```python
from build123d import *

# Parameters (mm, degrees)
SKETCH1_R           = 13.75
BOSS_EXTRUDE1_DEPTH = 6
SHELL1_T            = -0.5
SKETCH3_R           = 5
BOSS_EXTRUDE2_DEPTH = 6
BOSS_EXTRUDE7_START = 2
SKETCH10_R          = 13.25
BOSS_EXTRUDE7_DEPTH = 2
BOSS_EXTRUDE3_START = 25.55
SKETCH4_R           = 13.75
BOSS_EXTRUDE3_DEPTH = 25.55
CHAMFER1_SIZE       = 2
SKETCH5_R           = 3.9
BOSS_EXTRUDE4_DEPTH = 4.8
SKETCH6_R           = 2.9
BOSS_EXTRUDE5_DEPTH = 4.2
CHAMFER2_SIZE       = 0.5
CUT_EXTRUDE1_START  = -5
CUT_EXTRUDE1_DEPTH  = 24.2
CUT_EXTRUDE2_START  = -5
CUT_EXTRUDE2_DEPTH  = 24.2
BOSS_EXTRUDE8_DEPTH = 6.687218579
BOSS_EXTRUDE8_DRAFT = 8


# Read off the part's stored shape, not the designer's step: Boss-Extrude8
with BuildPart() as part:
    # Sketch1 → Boss-Extrude1 (new body)
    with BuildSketch(Plane.XY):
        Circle(SKETCH1_R)
    extrude(amount=BOSS_EXTRUDE1_DEPTH)

    # Shell1
    shell1_openings = [part.faces().sort_by_distance(p)[0] for p in [
        (0, 0, 0),
    ]]
    offset(amount=SHELL1_T, openings=shell1_openings, kind=Kind.INTERSECTION)

    # Sketch3 → Boss-Extrude2 (add)
    with BuildSketch(Plane(origin=(0, 0, 5.5), x_dir=(-1, 0, 0), z_dir=(0, 0, -1))):
        with Locations(Location((0, 0, 0), (0, 0, 180))):
            Circle(SKETCH3_R)
    extrude(amount=BOSS_EXTRUDE2_DEPTH)

    # Sketch10 → Boss-Extrude7 (add)
    with BuildSketch(Plane(origin=(0, 0, 5.5), x_dir=(-1, 0, 0), z_dir=(0, 0, -1)).offset(BOSS_EXTRUDE7_START)):
        Circle(SKETCH10_R)
    extrude(amount=-BOSS_EXTRUDE7_DEPTH)

    # Sketch4 → Boss-Extrude3 (add)
    with BuildSketch(Plane(origin=(0, 0, -0.5), x_dir=(-1, 0, 0), z_dir=(0, 0, -1)).offset(BOSS_EXTRUDE3_START)):
        with Locations(Location((0, 0, 0), (0, 0, 180))):
            Circle(SKETCH4_R)
    extrude(amount=-BOSS_EXTRUDE3_DEPTH)

    # Chamfer1
    chamfer1_edges = [part.edges().sort_by_distance(p)[0] for p in [
        (-13.75, 0, -26.05),
    ]]
    chamfer(chamfer1_edges, length=CHAMFER1_SIZE)

    # Sketch5 → Boss-Extrude4 (add)
    with BuildSketch(Plane(origin=(0, 0, -26.05), x_dir=(-1, 0, 0), z_dir=(0, 0, -1))):
        Circle(SKETCH5_R)
    extrude(amount=BOSS_EXTRUDE4_DEPTH)

    # Sketch6 → Boss-Extrude5 (add)
    with BuildSketch(Plane(origin=(0, 0, -30.85), x_dir=(-1, 0, 0), z_dir=(0, 0, -1))):
        Circle(SKETCH6_R)
    extrude(amount=BOSS_EXTRUDE5_DEPTH)

    # Chamfer2
    chamfer2_edges = [part.edges().sort_by_distance(p)[0] for p in [
        (2.9, 0, -35.05),
    ]]
    chamfer(chamfer2_edges, length=CHAMFER2_SIZE)

    # Sketch7 → Cut-Extrude1 (cut)
    with BuildSketch(Plane(origin=(0, 0, 0), x_dir=(0, 0, -1), z_dir=(1, 0, 0)).offset(CUT_EXTRUDE1_START)):
        with BuildLine():
            Line((-4, -5), (-4, 5))
            ThreePointArc((-4, 5), (-2.5, 6.5), (-1, 5))
            Line((-1, 5), (-1, -5))
            ThreePointArc((-1, -5), (-2.5, -6.5), (-4, -5))
        make_face()
    extrude(amount=-CUT_EXTRUDE1_DEPTH, mode=Mode.SUBTRACT)

    # Sketch8 → Cut-Extrude2 (cut)
    with BuildSketch(Plane(origin=(0, 0, 0), x_dir=(1, 0, 0), z_dir=(0, 1, 0)).offset(CUT_EXTRUDE2_START)):
        with BuildLine():
            Line((-5, -1), (5, -1))
            ThreePointArc((5, -1), (6.5, -2.5), (5, -4))
            Line((5, -4), (-5, -4))
            ThreePointArc((-5, -4), (-6.5, -2.5), (-5, -1))
        make_face()
    cut_extrude2 = extrude(amount=-CUT_EXTRUDE2_DEPTH, mode=Mode.SUBTRACT)

    # Mirror1: Cut-Extrude2 across plane
    add(cut_extrude2.mirror(Plane.ZX), mode=Mode.SUBTRACT)


with BuildPart() as boss_extrude8_tool:
    # Boss-Extrude8 outline → Boss-Extrude8 (with draft: the straight prism first)
    with BuildSketch(Plane(origin=(20, 0, 0), x_dir=(0, 0, -1), z_dir=(1, 0, 0))):
        with BuildLine():
            ThreePointArc((-3.5, -1.5), (-2.5, -2.5), (-1.5, -1.5))
            Line((-1.5, -1.5), (-1.5, 1.5))
            ThreePointArc((-1.5, 1.5), (-2.5, 2.5), (-3.5, 1.5))
            Line((-3.5, 1.5), (-3.5, -1.5))
        make_face()
    extrude(amount=-BOSS_EXTRUDE8_DEPTH)
    # Boss-Extrude8: the draft: its side faces are tilted about the plane it starts from
    boss_extrude8_sides = [boss_extrude8_tool.faces().sort_by_distance(p)[0] for p in [
        (16.656390711, 0, 3.5),
        (16.65639071, -2.5, 2.5),
        (16.656390711, 0, 1.5),
        (16.65639071, 2.5, 2.5),
    ]]
    draft(boss_extrude8_sides, Plane(origin=(20, 0, 0), x_dir=(0, 0, -1), z_dir=(1, 0, 0)), BOSS_EXTRUDE8_DRAFT)


with BuildPart() as part_1:
    add(part.part)

    # Boss-Extrude8: add boss_extrude8_tool
    add(boss_extrude8_tool.part)


solid = part_1.part
```
Work out the finished part from the listing and answer in its coordinate system (mm). A direction names the side the tool comes from. Round coordinates to 2 decimals unless told otherwise and drop trailing zeros. Loops run counter-clockwise (first coordinate to the right, second up) from the corner with the lowest first, then second, coordinate; pieces in that order, holes last. Notation, with made-up numbers: M 52.25,44.25 L 98.25,44.25 A29 ccw 98.25,67.25 Z; hole C 48.5,13 d10. An arc over 180 degrees is marked long. Use CSV: the item, a comma, the result in double quotes.
Q1. A tool of negligible diameter and unlimited length cuts with its end or side. For faces 1 (the flat face through (-13.4, 0, 1)), 2 (the flat face through (8, 0, 3.5)), 3 (the flat face through (-3, -3, -26.05)), 4 (the flat face through (0, 13.4, 1)), 5 (the cylindrical face through (5.9, -9.5, 3.7)), from which of +Z, -Z, +X, -X, +Y, -Y can it reach the whole face along a straight path? Write none if from no direction.
Determined:
face 1,"-X"
face 2,"none"
face 3,"-Z"
face 4,"+Y"
face 5,"-Y"
Q2. Section A-A, the plane z = -31.5 is taken. Determine the outline of the cut face in (x, y).
Determined:
outline,"C 0,0 d5.8"
Q3. Section B-B, the plane x = 16.5 is taken. Determine the outline of the cut face in (y, z), then the cut area to 3 significant figures.
Determined:
outline,"M -1.5,1.01 L 1.5,1.01 A1.49 ccw 1.5,3.99 L -1.5,3.99 A1.49 ccw Z"
area,"15.9 mm2"
Q4. Consider L1, parallel to Z at x = -3.5, y = -3.75; L2, parallel to Z at x = 3.5, y = -9.5; L3, parallel to Y at x = 0, z = -29. Determine where each line is inside the solid, lowest interval first.
Determined:
L1,"-26.05 to -0.5, 3.5 to 6"
L2,"-26.05 to -0.5, 4 to 6"
L3,"-3.9 to 3.9"
Q5. Section C-C, the plane z = -2 is taken. Determine the outline of the cut face in (x, y).
Determined:
outline,"C 0,0 d27.5"
Q6. Each of these flat-tipped pins is pushed along its axis until it touches: pin 1 (5.5 mm diameter, centred on x = -3, y = -3, fed in from -Z); pin 2 (10 mm diameter, centred on x = 5.5, z = -30.5, fed in from -Y); pin 3 (2 mm diameter, centred on y = -8.5, z = -4, fed in from +X); pin 4 (7 mm diameter, centred on x = -2, y = 9.5, fed in from -Z). Where does it stop, or does it pass through?
Determined:
pin 1,"z = -35.05"
pin 2,"y = -11.39"
pin 3,"x = 11.52"
pin 4,"z = -26.05"
Q7. The mould has two halves that part along Z. Classify faces 6 (the cylindrical face through (-9.754, -5.76, 3.794)), 7 (the flat face through (0, 0, -35.05)), 8 (the flat face through (0, 0, 6)): pulls with the +Z half, pulls with the -Z half, needs draft (parallel to the pull), parting line crosses it, or undercut.
Determined:
face 6,"undercut"
face 7,"pulls with the -Z half"
face 8,"pulls with the +Z half"
